Build history of the part. All positions in model axes, mm. Face numbers are marked on the shaded views. Coordinates: 2 decimals unless noted, no trailing zeros. Write each loop counter-clockwise with the first axis right and the second up, starting at its lowest first coordinate (ties: lowest second). Pieces come first, ordered by that corner, then holes.
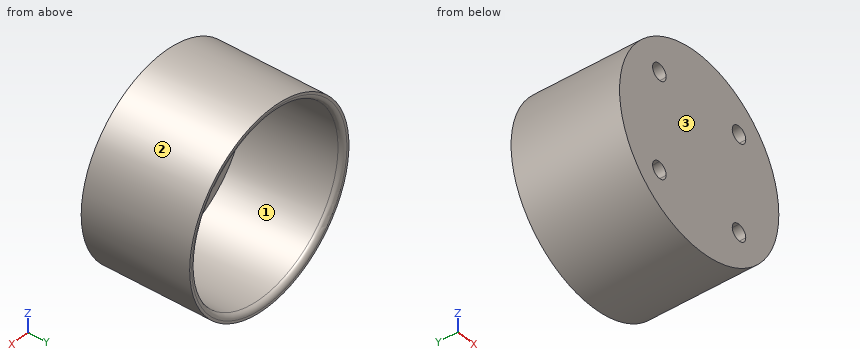
```python
from build123d import *

# Parameters (mm, degrees)
CUT_EXTRUDE_1_DEPTH = 10


with BuildPart() as part:
    # 草图3 → 旋转1 (revolve)
    with BuildSketch(Plane.XY):
        with BuildLine():
            Line((0, 0), (0, 2))
            Line((0, 2), (18.5, 2))
            Line((18.5, 2), (18.5, 21))
            ThreePointArc((18.5, 21), (18.792893219, 21.707106781), (19.5, 22))
            Line((19.5, 22), (20, 22))
            Line((20, 22), (20, 2))
            Line((20, 2), (20, 1))
            Line((20, 1), (20, 0))
            Line((20, 0), (0, 0))
        make_face()
    revolve(axis=Axis((0, 0, 0), (0, 1, 0)))

    # 草图4 → 切除-拉伸1 (cut)
    with BuildSketch(Plane(origin=(0, 2, 0), x_dir=(1, 0, 0), z_dir=(0, 1, 0))):
        with BuildLine():
            ThreePointArc((10, -8.3), (8.797918472, -8.797918472), (8.3, -10))
            Line((8.3, -10), (10, -10))
            Line((10, -10), (10, -8.3))
        make_face()
        with BuildLine():
            Line((10, -10), (8.3, -10))
            ThreePointArc((8.3, -10), (10, -11.7), (11.7, -10))
            ThreePointArc((11.7, -10), (11.202081528, -8.797918472), (10, -8.3))
            Line((10, -8.3), (10, -10))
        make_face()
        with BuildLine():
            ThreePointArc((-10, -8.3), (-11.202081528, -11.202081528), (-8.3, -10))
            Line((-8.3, -10), (-10, -10))
            Line((-10, -10), (-10, -8.3))
        make_face()
        with BuildLine():
            Line((-10, -10), (-8.3, -10))
            ThreePointArc((-8.3, -10), (-8.797918472, -8.797918472), (-10, -8.3))
            Line((-10, -8.3), (-10, -10))
        make_face()
        with BuildLine():
            ThreePointArc((-8.3, 10), (-11.202081528, 11.202081528), (-10, 8.3))
            Line((-10, 8.3), (-10, 10))
            Line((-10, 10), (-8.3, 10))
        make_face()
        with BuildLine():
            Line((-10, 10), (-10, 8.3))
            ThreePointArc((-10, 8.3), (-8.797918472, 8.797918472), (-8.3, 10))
            Line((-8.3, 10), (-10, 10))
        make_face()
        with BuildLine():
            ThreePointArc((8.3, 10), (8.797918472, 8.797918472), (10, 8.3))
            Line((10, 8.3), (10, 10))
            Line((10, 10), (8.3, 10))
        make_face()
        with BuildLine():
            Line((10, 10), (10, 8.3))
            ThreePointArc((10, 8.3), (11.202081528, 8.797918472), (11.7, 10))
            ThreePointArc((11.7, 10), (10, 11.7), (8.3, 10))
            Line((8.3, 10), (10, 10))
        make_face()
    extrude(amount=-CUT_EXTRUDE_1_DEPTH, mode=Mode.SUBTRACT)


solid = part.part
```
1. Probe line 1 along Z through (x, y) = (0, 10.75); line 2 along X through (y, z) = (0.85, 10). List the from-to ranges inside material, lowest first.
Computed values:
line 1: z = -20 to -18.5, 18.5 to 20
line 2: x = -17.32 to -11.7, -8.3 to 8.3, 11.7 to 17.32
2. Saw through at A-A on x = 0. List the corners of the cut face in (y, z), plus the area to 3 significant figures.
Computed values:
outline: (0, -20) - (22, -20) - (22, -19.5) arc R1 ccw to (21, -18.5) - (2, -18.5) - (2, 18.5) - (21, 18.5) arc R1 ccw to (22, 19.5) - (22, 20) - (0, 20) - close
area: 140 mm2
3. Saw through at C-C on y = 15.75. List the corners of the cut face in (x, z).
Computed values:
outline: circle Ø40 at (0, 0); hole circle Ø37 at (0, 0)
4. Flat gauge pins, fed straight in: pin 1 (2 mm diameter, centred on x = 10, z = -9.5, fed in from -Y); pin 2 (1 mm diameter, centred on y = 15, z = 7, fed in from -X); pin 3 (5 mm diameter, centred on x = -8.5, z = 6.5, fed in from +Y); pin 4 (12 mm diameter, centred on y = 17.5, z = -8.5, fed in from -X). Where does each tip first touch, or does it go through?
Computed values:
pin 1: passes through
pin 2: stops at x = -18.91
pin 3: stops at y = 2
pin 4: stops at x = -19.84
5. Saw through at D-D on x = 11. State how many separate pieces and enclosed holes the cut face has, plus the area to 3 significant figures.
Computed values:
separate pieces: 3
enclosed holes: 0
area: 128 mm2
6. Mould opens along X. For the marked faces 1, 2 and 3 say: +X half, -X half, draft (parallel to the pull), parting line (faces both ways), or undercut.
Computed values:
face 1: undercut
face 2: parting line
face 3: draft
7. Saw through at B-B on z = 0. List the corners of the cut face in (x, y).
Computed values:
outline: (-20, 0) - (20, 0) - (20, 22) - (19.5, 22) arc R1 ccw to (18.5, 21) - (18.5, 2) - (-18.5, 2) - (-18.5, 21) arc R1 ccw to (-19.5, 22) - (-20, 22) - close
